Could you check a few things on this drawing? It's one solid part, dimensions in mm from its lowest x, y, z. A direction names the side the tool comes from. Give positions to 0.01 mm unless a question says otherwise; leave off trailing zeros. Order: outer loops, then holes, each group sorted by start corner. A loop starts at its lowest first (then second) coordinate and runs counter-clockwise, first axis right, second up. Notation, with made-up numbers: (-16.75, 56) - (32.25, 56) arc R22 ccw to (32.25, 70) - close; hole circle Ø11 at (48.25, 70). An arc over 180 degrees is marked (long way). Answer as CSV lines item,"result".
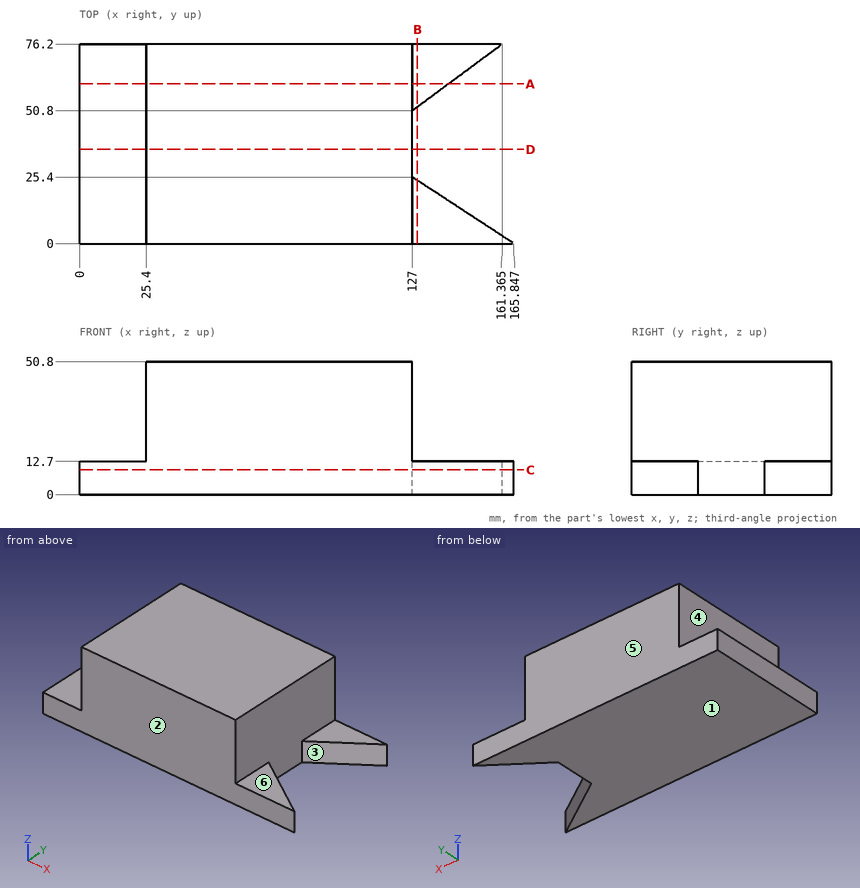
1) I want a section at C-C on z = 9.5. Write out the boundary of the cut face in (x, y) (1 decimal).
Answer block:
outline,"(0, 0) - (165.8, 0) - (127, 25.4) - (127, 50.8) - (161.4, 76.2) - (0, 76.2) - close"
2) If we mould it in two halves opening along Y, with no side actions, what happens to the marked faces 1, 2 and 3? For each: +Y half, -Y half, draft (parallel to the pull), parting line (faces both ways), or undercut.
Answer block:
face 1,"draft"
face 2,"-Y half"
face 3,"undercut"
3) I need wall thicknesses on line 1 along Z through (x, y) = (7.5, 67.5); line 2 along X through (y, z) = (8.5, 17.5); line 3 along X through (y, z) = (29, 9). Which ranges of each line are inside material? Lowest first, please. Write a range as [from, to].
Answer block:
line 1,"[0, 12.7]"
line 2,"[25.4, 127]"
line 3,"[0, 127]"
4) I want a section at B-B on x = 129. Write out the boundary of the cut face in (y, z).
Answer block:
outline,"(0, 0) - (24.09, 0) - (24.09, 12.7) - (0, 12.7) - close; (52.28, 0) - (76.2, 0) - (76.2, 12.7) - (52.28, 12.7) - close"
5) I'm going to push flat-ended pins straight in: P1, Ø20.5, axis at x = 144, y = 9, coming from the +Z side; P2, Ø10, axis at y = 53, z = 22.5, coming from the +X side; P3, Ø8, axis at y = 41.5, z = 20.5, coming from the -X side. Where does each tip first touch, or does it pass through?
Answer block:
P1,"z = 12.7"
P2,"x = 127"
P3,"x = 25.4"
6) Which directions (+Z, -Z, +X, -X, +Y, -Y) give clear straight access to the entire face, cutting with the end or side of a thin tool? Please do the marked faces 4, 5 and 6.
Answer block:
face 4,"+Z, -X, +Y, -Y"
face 5,"+Z, -Z, +X, -X, +Y"
face 6,"+Z, +X, +Y, -Y"
7) I want a section at A-A on y = 61. Write out the boundary of the cut face in (x, z).
Answer block:
outline,"(0, 0) - (140.8, 0) - (140.8, 12.7) - (127, 12.7) - (127, 50.8) - (25.4, 50.8) - (25.4, 12.7) - (0, 12.7) - close"
8) I want a section at D-D on y = 36. Write out the boundary of the cut face in (x, z).
Answer block:
outline,"(0, 0) - (127, 0) - (127, 50.8) - (25.4, 50.8) - (25.4, 12.7) - (0, 12.7) - close"
